Autodesk Inventor part; units mm, degrees
ref_plane "YZ Plane" through (0, 0, 0) normal (1, 0, 0) x (0, 1, 0)
ref_plane "XZ Plane" through (0, 0, 0) normal (0, 1, 0) x (-1, 0, 0)
ref_plane "XY Plane" through (0, 0, 0) normal (0, 0, 1) x (1, 0, 0)
sketch "Skizze1" plane through (0, 0, 0) normal (1, 0, 0) x (0, 1, 0)
  line L0 (6, 0) -> (30, 0)
  line L1 (30, 0) -> (30, 11)
  line L2 (9, 27) -> (9, 9)
  line L3 (9, 27) -> (22, 27)
  line L4 (22, 27) -> (22, 11)
  line L5 (30, 11) -> (22, 11)
  circle A0 centre (15.5, 15) radius 0.5
  circle A1 centre (14.5, 20.5) radius 0.5
  circle A2 centre (27, 8) radius 0.5
  line L6 (0, 32.4) -> (0, -5.4)
  line L7 (1.2, 0) -> (34.8, 0)
  line L8 (9, 9) -> (6, 6)
  line L9 (6, 6) -> (6, 0)
  circle A3 centre (14.5, 11) radius 0.5
  line L10 (14.5, 20.5) -> (14.5, 11) construction
  dimension "d1" = 11
  dimension "d3" = 27
  dimension "d21" = 1
  dimension "d28" = 1
  dimension "d41" = 1
  dimension "d43" = 8
  dimension "d54" = 9
  dimension "d55" = 27
  dimension "d61" = 15
  dimension "d62" = 15.5
  dimension "d127" = 30
  dimension "d172" = 6
  dimension "d175" = 6
  dimension "d176" = 45
  dimension "d180" = 22
  dimension "d197" = 1
  dimension "d198" = 14.5
  dimension "d199" = 11
  dimension "d201" = 9.5
  dimension "d202" = 0
extrude "Extrusion1" add sketch "Skizze1" along normal mid plane 6
sketch "Skizze9" plane through (-3, 0, 0) normal (-1, 0, 0) x (0, 0, 1)
  circle A0 centre (8, 27) radius 0.5
  point P0 (0, 0)
hole "Feder" at (-3, 27, 8) direction (1, 0, 0) diameter 2.459 end through all
sketch "Skizze3" plane through (-3, 0, 0) normal (-1, 0, 0) x (0, 0, 1)
  circle A0 centre (20.5, 14.5) radius 0.5
  circle A1 centre (11, 14.5) radius 0.5
hole "Dribbler" at (-3, 14.5, 20.5) at (-3, 14.5, 11) direction (1, 0, 0) diameter 2.459 end through all
sketch "Skizze4" plane through (-3, 0, 0) normal (-1, 0, 0) x (0, 0, 1)
  circle A0 centre (15, 15.5) radius 0.5
  circle A1 centre (15, 15.5) radius 0.5
  point P0 (0, 0)
hole "Chipper" at (-3, 15.5, 15) direction (1, 0, 0) diameter 4 end through all
sketch "Skizze5" plane through (3, 30, 0) normal (0, 0, -1) x (-1, 0, 0)
  line L0 (6, 0) -> (0, 0)
  line L1 (0, -24) -> (0, 0)
  line L2 (6, 0) -> (6, -24)
  line L3 (3, -24) -> (3, 0) construction
  line L4 (6, -24) -> (0, -24)
  line L5 (-1.2, -30) -> (7.2, -30)
  point P0 (3, -20.5)
  point P1 (3, -6.5)
  point P2 (3, -13.5)
  point P3 (3, -12)
  dimension "d58" = 7
  dimension "d89" = 7
  dimension "d185" = 9.5
hole "Montage" at (0, 9.5, 0) at (0, 23.5, 0) direction (0, 0, 1) diameter 2.459 depth 7 tip angle 118
fillet "Rundung2" radius 3 4 edges at (0, 22, 11) (0, 30, 11) (0, 9, 9) (0, 6, 6)
sketch "Skizze16" plane through (-3, 0, 0) normal (-1, 0, 0) x (0, 0, 1)
  line L0 (2.5, 27) -> (2.5, 17) construction
  line L1 (0, 36) -> (0, -6) construction
  point P0 (0, 0)
  dimension "d161" = 17
  dimension "d162" = 10
  dimension "d177" = 2.5
hole "Bohrung10" at (-3, 27, 2.5) at (-3, 17, 2.5) direction (1, 0, 0) diameter 2 end through all
fillet "Rundung7" radius 5 1 edges at (0, 9, 27)
fillet "Rundung8" radius 2 1 edges at (0, 22, 27)
properties part number "Dribbler Lagerbock v2" material "Aluminium 6061"
The model under review builds one solid part; all positions refer to its coordinate system, in mm. A direction names the side the tool comes from. Give positions to 0.01 mm unless a question says otherwise; leave off trailing zeros. Loops run counter-clockwise (first coordinate to the right, second up) from the corner with the lowest first, then second, coordinate; pieces in that order, holes last. Notation, with made-up numbers: (30, 79) -> (69, 79) arc R26 ccw to (69, 114) -> close; hole circle Ø4 at (-24, 14). An arc over 180 degrees is marked (long way). Answer as a JSON object with one key per item and string values. Group by question number.
Q1. Insertion check: pin 1 (1.8 mm diameter, centred on x = 1.5, z = 15.5, fed in from -Y); pin 2 (3 mm diameter, centred on x = 0, y = 9.5, fed in from +Z); pin 3 (0.6 mm diameter, centred on x = 1.5, y = 26, fed in from +Z); pin 4 (1.2 mm diameter, centred on y = 27, z = 2.5, fed in from +X) (1 decimal). Each pin has a flat end and moves straight along its axis. Give the tip position at first contact, or say it passes through.
Q2. Take a section at B-B (z = 2.5). Write out the cut boundary in (x, y), plus the area to 3 significant figures.
Q3. Wall thickness on line 1 along Z through (x, y) = (-0.2, 27); line 2 along Y through (x, z) = (1.4, 8); line 3 along Z through (x, y) = (0.1, 14.5): over which ranges is each line inside the solid? List them lowest first.
Q4. Take a section at C-C (z = 20.5). Write out the cut boundary in (x, y).
Q5. Take a section at D-D (x = 0.55). State how many separate pieces and enclosed holes the cut face has, plus the area to 3 significant figures.
Q6. Draft analysis for pull direction Y (two halves, no side actions). For faces 4 (the cylindrical face through (-0.04, 6.22, 5.89)), 5 (the flat face through (0, 17, 27)), 6 (the cylindrical face through (0.04, 29.14, 10.1)), 7 (the cylindrical face through (0.04, 28.2, 7.73)), state which applies: pulls with the +Y half, pulls with the -Y half, needs draft (parallel to the pull), parting line crosses it, or undercut.
Q7. Take a section at A-A (z = 15). Write out the cut boundary in (x, y).
Q8. Tool access review of faces 1 (the cylindrical face through (0.471, 24.636, 3.549)), 2 (the flat face through (0, 26, 11)), 3 (the flat face through (0, 9, 16)): name each direction out of +Z, -Z, +X, -X, +Y, -Y from which nothing blocks a thin tool from reaching the whole face with its end or side.
Answer below:
{
 "1": {"pin 1": "stops at y = 9", "pin 2": "stops at z = 26", "pin 3": "stops at z = 11", "pin 4": "passes through"},
 "2": {"outline": "(-3, 6) -> (3, 6) -> (3, 16) -> (-3, 16) -> close; (-3, 18) -> (3, 18) -> (3, 26) -> (-3, 26) -> close; (-3, 28) -> (3, 28) -> (3, 30) -> (-3, 30) -> close; hole circle Ø2.46 at (0, 9.5); hole circle Ø2.46 at (0, 23.5)", "area": "111 mm2"},
 "3": {"line 1": "z = 0 to 1.5, 3.5 to 6.77, 9.23 to 11", "line 2": "y = 8 to 25.77, 28.23 to 30", "line 3": "z = 0 to 9.77, 12.23 to 13.27, 16.73 to 19.27, 21.73 to 27"},
 "4": {"outline": "(-3, 9) -> (3, 9) -> (3, 13.27) -> (-3, 13.27) -> close; (-3, 15.73) -> (3, 15.73) -> (3, 22) -> (-3, 22) -> close"},
 "5": {"separate pieces": "1", "enclosed holes": "6", "area": "390 mm2"},
 "6": {"face 4": "pulls with the -Y half", "face 5": "needs draft", "face 6": "pulls with the +Y half", "face 7": "undercut"},
 "7": {"outline": "(-3, 9) -> (3, 9) -> (3, 13.5) -> (-3, 13.5) -> close; (-3, 17.5) -> (3, 17.5) -> (3, 22) -> (-3, 22) -> close"},
 "8": {"face 1": "-Z", "face 2": "+Z, +X, -X, +Y", "face 3": "+Z, +X, -X, -Y"}
}
